Read the model definition and answer for the solid it produces. Units are mm, in the model's axes. Give positions to 0.01 mm unless a question says otherwise; leave off trailing zeros. Order: outer loops, then holes, each group sorted by start corner. A loop starts at its lowest first (then second) coordinate and runs counter-clockwise, first axis right, second up. Notation, with made-up numbers: (71, 60.5) - (108, 60.5) arc R11 ccw to (108, 79.5) - close; hole circle Ø3 at (-14.5, 76.25). An arc over 180 degrees is marked (long way). Use a Markdown table: item, result. Add a question column.
1. A cutting plane is placed at A-A on y = 7.5. Determine the outline of the cut face in (x, z), and give its area (3 significant figures).
2. A flat-ended cylindrical pin translates along its axis: P1, Ø8, axis at x = 91, z = 30, coming from the +Y side. Find the tip coordinate at first contact, or state that the pin passes through.
3. A cutting plane is placed at C-C on x = 86. Determine the outline of the cut face in (y, z), and give its area (3 significant figures).
4. A cutting plane is placed at B-B on z = 53.5. Determine the outline of the cut face in (x, y).
5. Consider L1, parallel to X at y = 7.5, z = 84.5; L2, parallel to Y at x = 112.5, z = 143.5; L3, parallel to Y at x = 33, z = 69.5. Determine where each line is inside the solid, lowest interval first.
```python
from build123d import *

# Parameters (mm, degrees)
SKETCH_1_R          = 5
EXTRUDE_1_DEPTH     = 210
SKETCH_2_R          = 7.5
CUT_EXTRUDE_1_DEPTH = 10
SKETCH_3_R          = 7.5
CUT_EXTRUDE_2_DEPTH = 10


with BuildPart() as part:
    # 草图1 → 凸台-拉伸1 (new body)
    with BuildSketch(Plane.XY):
        with BuildLine():
            Line((105.428932188, 5), (100.074072144, 5))
            Line((100.074072144, 5), (1, 5))
            ThreePointArc((1, 5), (0.292893219, 4.707106781), (0, 4))
            Line((0, 4), (0, 1))
            ThreePointArc((0, 1), (0.292893219, 0.292893219), (1, 0))
            Line((1, 0), (112.5, 0))
            ThreePointArc((112.5, 0), (116.830127019, 13.623724357), (105.428932188, 5))
        make_face()
        with Locations((112.5, 7.5)):
            Circle(SKETCH_1_R, mode=Mode.SUBTRACT)
    extrude(amount=EXTRUDE_1_DEPTH)

    # 草图2 → 切除-拉伸1 (cut)
    with BuildSketch(Plane.XY.offset(210)):
        with Locations((112.5, 7.5)):
            Circle(SKETCH_2_R)
    extrude(amount=-CUT_EXTRUDE_1_DEPTH, mode=Mode.SUBTRACT)

    # 草图3 → 切除-拉伸2 (cut)
    with BuildSketch(Plane(origin=(0, 0, 0), x_dir=(-1, 0, 0), z_dir=(0, 0, -1))):
        with Locations((-112.5, 7.5)):
            Circle(SKETCH_3_R)
    extrude(amount=-CUT_EXTRUDE_2_DEPTH, mode=Mode.SUBTRACT)


solid = part.part
```
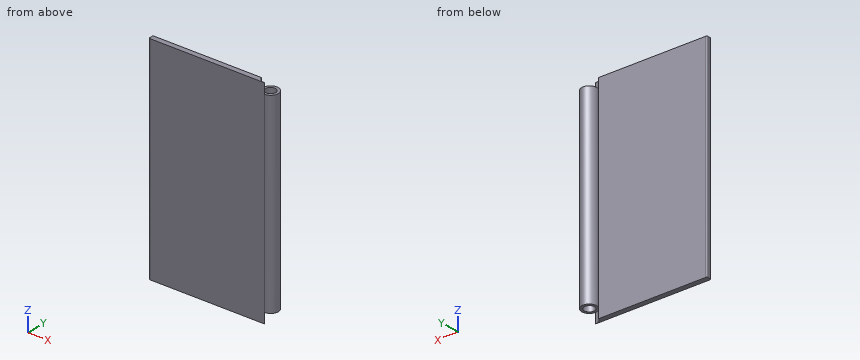
Output values:
| question | item | result |
|---|---|---|
| 1 | outline | (105, 10) - (107.5, 10) - (107.5, 200) - (105, 200) - close; (117.5, 10) - (120, 10) - (120, 200) - (117.5, 200) - close |
| 1 | area | 950 mm² |
| 2 | P1 | y = 5 |
| 3 | outline | (0, 0) - (5, 0) - (5, 210) - (0, 210) - close |
| 3 | area | 1,050 mm² |
| 4 | outline | (0, 1) arc R1 ccw to (1, 0) - (112.5, 0) arc R7.5 ccw (long way) to (105.43, 5) - (1, 5) arc R1 ccw to (0, 4) - close; hole circle Ø10 at (112.5, 7.5) |
| 5 | L1 | 105 to 107.5, 117.5 to 120 |
| 5 | L2 | 0 to 2.5, 12.5 to 15 |
| 5 | L3 | 0 to 5 |
